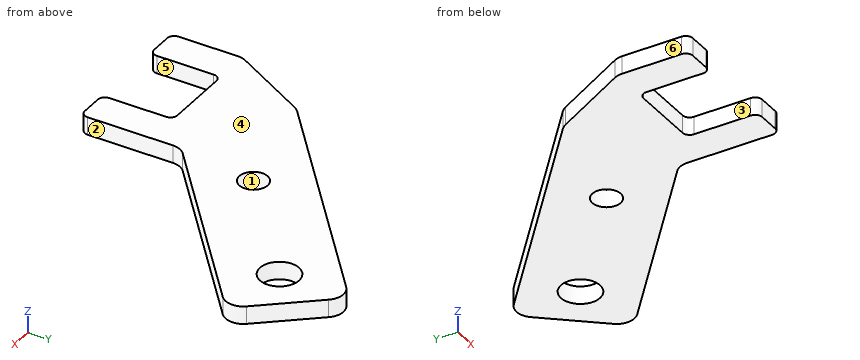
```python
from build123d import *

# Parameters (mm, degrees)
ESQUISSE1_R        = 5.5
ESQUISSE1_R_2      = 4
BOSS_EXTRU_1_DEPTH = 5
CONG_1_R           = 5
CONG_2_R           = 2


with BuildPart() as part:
    # Esquisse1 → Boss.-Extru.1 (new body)
    with BuildSketch(Plane.XY):
        Polygon((34.397799289, 8.390996312), (89.511576954, 54.636946823), (70.227948663, 77.618280117), (5.114170998, 22.981333294), (-7.602200711, 0), (-7.602200711, -20), (2.397799289, -20), (2.397799289, 0), (24.397799289, 0), (24.397799289, -20), (34.397799289, -20), align=None)
        with Locations((69.911185048, 57.771374544)):
            Circle(ESQUISSE1_R, mode=Mode.SUBTRACT)
        with Locations((37.737318437, 30.774294937)):
            Circle(ESQUISSE1_R_2, mode=Mode.SUBTRACT)
    extrude(amount=BOSS_EXTRU_1_DEPTH)

    # Congé1
    cong_1_edges = [part.edges().sort_by_distance(p)[0] for p in [
        (-7.602200711, 0, 2.5),
        (5.114170998, 22.981333294, 2.5),
        (70.227948663, 77.618280117, 2.5),
        (89.511576954, 54.636946823, 2.5),
        (34.397799289, 8.390996312, 2.5),
    ]]
    fillet(cong_1_edges, radius=CONG_1_R)

    # Congé2
    cong_2_edges = [part.edges().sort_by_distance(p)[0] for p in [
        (2.397799289, 0, 2.5),
        (2.397799289, -20, 2.5),
        (-7.602200711, -20, 2.5),
        (34.397799289, -20, 2.5),
        (24.397799289, -20, 2.5),
        (24.397799289, 0, 2.5),
    ]]
    fillet(cong_2_edges, radius=CONG_2_R)


solid = part.part
```
Check sheet for the modelled part. Datum: model origin and axes. Units: mm. Face numbers are marked on the shaded views. A direction names the side the tool comes from. Round coordinates to 2 decimals unless told otherwise and drop trailing zeros. Write each loop counter-clockwise with the first axis right and the second up, starting at its lowest first coordinate (ties: lowest second). Pieces come first, ordered by that corner, then holes. Notation, with made-up numbers: (-1.5, 37.5) -> (12.5, 37.5) arc R26 cw to (12.5, 69.5) -> close; hole circle Ø10 at (29, 73.25). An arc over 180 degrees is marked (long way). One line per question, with ' | ' between items. Start each with the question number.
1. Depth check by flat-ended pin: pin 1 (2 mm diameter, centred on y = 10, z = 2.5, fed in from -X); pin 2 (1 mm diameter, centred on y = 23.5, z = 4, fed in from +X); pin 3 (1.5 mm diameter, centred on x = 11.5, z = 0.5, fed in from -Y). Enter the tip coordinate at first touch or a pass-through.
2. Release check for a two-part mould opening along X. For the marked faces 4, 5 and 6 record: +X half, -X half, draft (parallel to the pull), parting line (faces both ways), or undercut.
3. Sectioned sample at D-D, the plane y = 13. Record the cut outline in (x, z), then the cut area to 3 significant figures.
4. Scan lines: line 1 along Y through (x, z) = (40.5, 2.9); line 2 along Y through (x, z) = (41, 2.25); line 3 along X through (y, z) = (38, 0.65). Record each from-to range of solid material in increasing order. Write a range as from..to.
5. Sectioned sample at B-B, the plane x = 70. Record the cut outline in (y, z), then the cut area to 3 significant figures.
6. Set-up check for the marked faces 1, 2 and 3: record each of +Z, -Z, +X, -X, +Y, -Y from which the full face is reachable in a straight line by a thin tool's end or side.
7. Sectioned sample at A-A, the plane y = 54. Record the cut outline in (x, z), then the cut area to 3 significant figures.
8. Sectioned sample at C-C, the plane z = 3.3. Record the cut outline in (x, y), then the cut area to 3 significant figures.
Taken from the geometry:
1) pin 1: stops at x = -2.62 | pin 2: stops at x = 53 | pin 3: stops at y = 0
2) face 4: draft | face 5: undercut | face 6: -X half
3) outline: (-0.41, 0) -> (39.89, 0) -> (39.89, 5) -> (-0.41, 5) -> close | area: 201 mm^2
4) line 1: y = 13.51..27.88, 33.67..52.67 | line 2: y = 13.93..28.46, 33.09..53.09 | line 3: x = 23.01..69.68
5) outline: (38.26, 0) -> (52.27, 0) -> (52.27, 5) -> (38.26, 5) -> close; (63.27, 0) -> (75.56, 0) -> (75.56, 5) -> (63.27, 5) -> close | area: 131 mm^2
6) face 1: +Z, -Z | face 2: +Z, -Z, +X, -Y | face 3: +Z, -Z, -Y
7) outline: (42.08, 0) -> (65.91, 0) -> (65.91, 5) -> (42.08, 5) -> close; (73.91, 0) -> (87.31, 0) -> (87.31, 5) -> (73.91, 5) -> close | area: 186 mm^2
8) outline: (-7.6, -18) arc R2 ccw to (-5.6, -20) -> (0.4, -20) arc R2 ccw to (2.4, -18) -> (2.4, -2) arc R2 cw to (4.4, 0) -> (22.4, 0) arc R2 cw to (24.4, -2) -> (24.4, -18) arc R2 ccw to (26.4, -20) -> (32.4, -20) arc R2 ccw to (34.4, -18) -> (34.4, 6.06) arc R5 cw to (36.18, 9.89) -> (85.68, 51.42) arc R5 ccw to (86.3, 58.47) -> (73.44, 73.79) arc R5 ccw to (66.4, 74.4) -> (5.83, 23.58) arc R5 ccw to (4.66, 22.17) -> (-6.98, 1.13) arc R5 ccw to (-7.6, -1.29) -> close; hole circle Ø8 at (37.74, 30.77); hole circle Ø11 at (69.91, 57.77) | area: 3,200 mm^2
